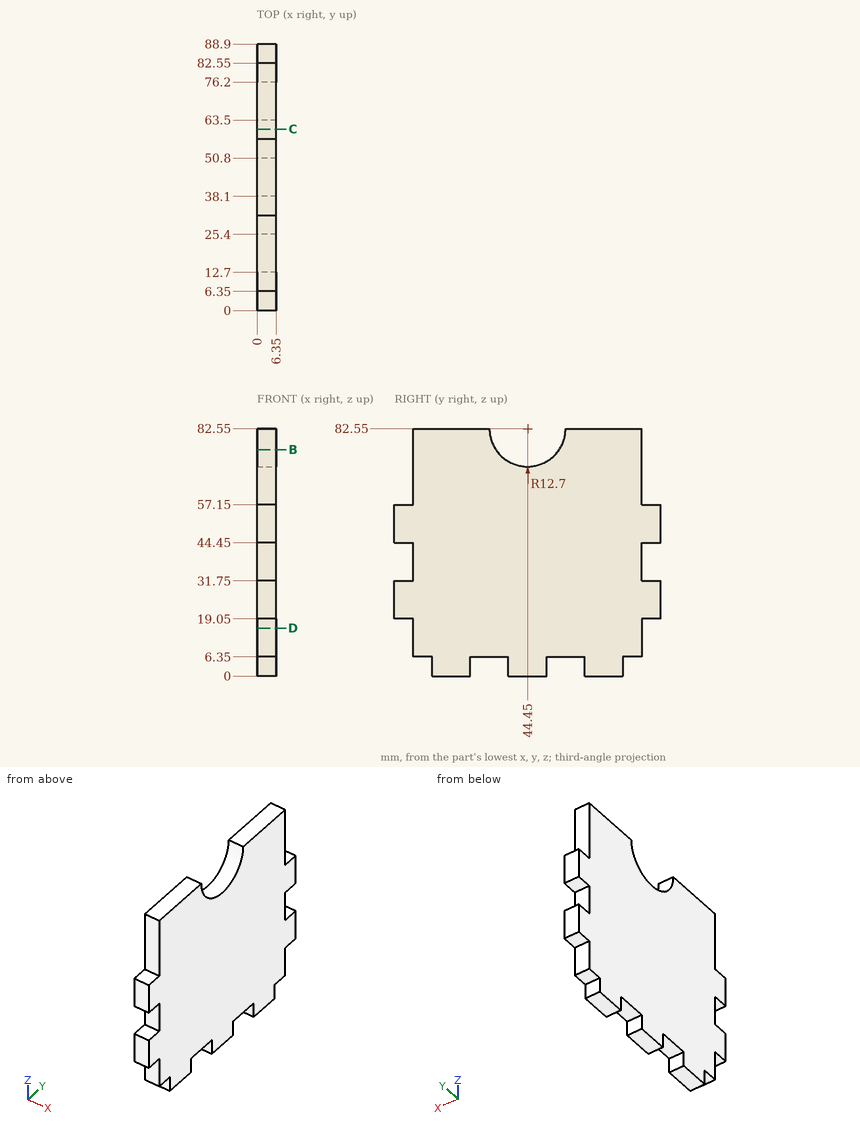
The drawing under review shows one solid part. Ordinate dimensions are in mm from its lowest x, y, z. Give positions to 0.01 mm unless a question says otherwise; leave off trailing zeros. Order: outer loops, then holes, each group sorted by start corner. A loop starts at its lowest first (then second) coordinate and runs counter-clockwise, first axis right, second up. Notation, with made-up numbers: (69.5, 2.25) - (94.5, 2.25) arc R30 cw to (94.5, 24.25) - close; hole circle Ø5 at (4.25, 5). An arc over 180 degrees is marked (long way). Answer as a JSON object with one key per item and string values. Group by question number.
Item 1: Wall thickness on line 1 along Y through (x, z) = (5.25, 6); line 2 along Y through (x, z) = (5.25, 36): over which ranges is each line inside the solid? List them lowest first.
Item 2: Take a section at B-B on z = 75.5. Give the boundary of the cut face in (x, y), and give its area (3 significant figures).
Item 3: Clearance check with flat-ended pins moving along their axes: pin 1 Ø1 at (x, z) = (1.5, 43.5) entering from +Y; pin 2 Ø3 at (x, z) = (2.5, 34) entering from -Y; pin 3 Ø3 at (x, y) = (2, 4.5) entering from +Z; pin 4 Ø1.5 at (y, z) = (38, 62) entering from -X. State where each tip first meets the part, or that it passes through.
Item 4: Take a section at C-C on y = 60.5. Give the boundary of the cut face in (x, z).
Reported:
{
 "1": {"line 1": "12.7 to 25.4, 38.1 to 50.8, 63.5 to 76.2", "line 2": "6.35 to 82.55"},
 "2": {"outline": "(0, 6.35) - (6.35, 6.35) - (6.35, 33.89) - (0, 33.89) - close; (0, 55.01) - (6.35, 55.01) - (6.35, 82.55) - (0, 82.55) - close", "area": "350 mm^2"},
 "3": {"pin 1": "y = 82.55", "pin 2": "y = 6.35", "pin 3": "z = 57.15", "pin 4": "x = 0"},
 "4": {"outline": "(0, 6.35) - (6.35, 6.35) - (6.35, 82.55) - (0, 82.55) - close"}
}
